Verification items for the finished model (mm, model axes). A direction names the side the tool comes from. Coordinates: 2 decimals unless noted, no trailing zeros. Write each loop counter-clockwise with the first axis right and the second up, starting at its lowest first coordinate (ties: lowest second). Pieces come first, ordered by that corner, then holes. Notation, with made-up numbers: M 74,83 L 122,83 A14 cw 122,110 Z; hole C 70.25,-13.5 d7. An arc over 180 degrees is marked long. Answer in a Markdown table with one row per item.
from build123d import *

# Parameters (mm, degrees)
SKETCH1_W             = 165.1
SKETCH1_H             = 152.4
BOSS_EXTRUDE1_DEPTH   = 12.7
BOSS_EXTRUDE2_DEPTH   = 12.7
CUT_EXTRUDE1_REACH    = 119.432
BOSS_EXTRUDE3_DEPTH   = 12.7
CUT_EXTRUDE2_DEPTH    = 12.7
F_8_CLEARANCE_HOLE1_D = 4.4958
SKETCH20_R            = 0.99187
CUT_EXTRUDE9_DEPTH    = 25.4
SKETCH21_R            = 3.175
SKETCH21_R_2          = 4.7625
CUT_EXTRUDE10_DEPTH   = 6.35


with BuildPart() as part:
    # Sketch1 → Boss-Extrude1 (new body)
    with BuildSketch(Plane.XY):
        Rectangle(SKETCH1_W, SKETCH1_H)
    extrude(amount=BOSS_EXTRUDE1_DEPTH)

    # Sketch2 → Boss-Extrude2 (add)
    with BuildSketch(Plane.XY.offset(12.7)):
        Polygon((-11.1125, 76.2), (11.1125, 76.2), (11.1125, 80.01), (10.664629469, 82.55), (-10.664629469, 82.55), (-11.1125, 80.01), align=None)
    extrude(amount=-BOSS_EXTRUDE2_DEPTH)

    # Sketch4 → Cut-Extrude1 (cut, up to next)
    with BuildSketch(Plane.XY.offset(12.7), mode=Mode.PRIVATE) as cut_extrude1_sk1:
        with BuildLine():
            Line((-17.7165, 76.2), (-11.1125, 76.2))
            ThreePointArc((-11.1125, 76.2), (-14.4145, 72.898), (-17.7165, 76.2))
        make_face()
    cut_extrude1_tool1 = extrude(cut_extrude1_sk1.sketch, amount=-CUT_EXTRUDE1_REACH, mode=Mode.PRIVATE) & part.part
    # Sketch4 → Cut-Extrude1 (cut, up to next)
    with BuildSketch(Plane.XY.offset(12.7), mode=Mode.PRIVATE) as cut_extrude1_sk2:
        with BuildLine():
            Line((11.1125, 76.2), (17.7165, 76.2))
            ThreePointArc((17.7165, 76.2), (14.4145, 72.898), (11.1125, 76.2))
        make_face()
    cut_extrude1_tool2 = extrude(cut_extrude1_sk2.sketch, amount=-CUT_EXTRUDE1_REACH, mode=Mode.PRIVATE) & part.part
    add(cut_extrude1_tool1.solids().sort_by_distance((-14.4145, 74.798588, 12.7))[0], mode=Mode.SUBTRACT)
    add(cut_extrude1_tool2.solids().sort_by_distance((14.4145, 74.798588, 12.7))[0], mode=Mode.SUBTRACT)

    # Sketch5 → Boss-Extrude3 (add)
    with BuildSketch(Plane.XY.offset(12.7)):
        Polygon((63.5, -76.2), (41.275, -76.2), (41.275, -80.01), (41.722870531, -82.55), (63.052129469, -82.55), (63.5, -80.01), align=None)
    boss_extrude3 = extrude(amount=-BOSS_EXTRUDE3_DEPTH)

    # Sketch6 → Cut-Extrude2 (cut)
    with BuildSketch(Plane.XY.offset(12.7)):
        with BuildLine():
            Line((34.671, -76.2), (41.275, -76.2))
            ThreePointArc((41.275, -76.2), (37.973, -72.898), (34.671, -76.2))
        make_face()
        with BuildLine():
            Line((63.5, -76.2), (70.104, -76.2))
            ThreePointArc((70.104, -76.2), (66.802, -72.898), (63.5, -76.2))
        make_face()
    cut_extrude2 = extrude(amount=-CUT_EXTRUDE2_DEPTH, mode=Mode.SUBTRACT)

    # Mirror1: Boss-Extrude3, Cut-Extrude2 across plane
    add(boss_extrude3.mirror(Plane(origin=(0, 0, 0), x_dir=(0, 0, 1), z_dir=(1, 0, 0))))
    add(cut_extrude2.mirror(Plane(origin=(0, 0, 0), x_dir=(0, 0, 1), z_dir=(1, 0, 0))), mode=Mode.SUBTRACT)

    # #8 Clearance Hole1 (through all)
    with Locations(Plane.XY.offset(12.7)):
        with Locations((0, -12.655936751), (63.5, 30.528732114), (-50.8, 30.528732114)):
            Hole(F_8_CLEARANCE_HOLE1_D / 2)

    # Sketch20 → Cut-Extrude9 (cut)
    with BuildSketch(Plane(origin=(82.55, 0, 0), x_dir=(0, 0, -1), z_dir=(1, 0, 0))):
        with Locations((-6.35, 0)):
            Circle(SKETCH20_R)
    cut_extrude9 = extrude(amount=-CUT_EXTRUDE9_DEPTH, mode=Mode.SUBTRACT)

    # Mirror3: Cut-Extrude9 across plane
    add(cut_extrude9.mirror(Plane(origin=(0, 0, 0), x_dir=(0, 0, 1), z_dir=(1, 0, 0))), mode=Mode.SUBTRACT)

    # Sketch21 → Cut-Extrude10 (cut)
    with BuildSketch(Plane(origin=(0, 0, 0), x_dir=(-1, 0, 0), z_dir=(0, 0, -1))):
        with Locations((0, -12.655936751)):
            Circle(SKETCH21_R)
        with Locations((-63.5, 30.528732114)):
            Circle(SKETCH21_R_2)
        with Locations((50.8, 30.528732114)):
            Circle(SKETCH21_R_2)
    extrude(amount=-CUT_EXTRUDE10_DEPTH, mode=Mode.SUBTRACT)


solid = part.part
1) Thickness scan on L1, parallel to Y at x = 71, z = 6.5; L2, parallel to Y at x = -74.5, z = 11.25; L3, parallel to Y at x = -9, z = 3.25. Record the ranges inside material, lowest first. Write a range as [from, to].
Response values:
| item | result |
|---|---|
| L1 | y = [-76.2, -0.98], [0.98, 76.2] |
| L2 | y = [-76.2, 76.2] |
| L3 | y = [-76.2, 82.55] |
2) Tool access check on faces 1 (the face through (-41.275, -78, 6)), 2 (the face through (68.258, 30.738, 3.131)), 3 (the face through (11.112, 78, 6)). Record the directions out of +Z, -Z, +X, -X, +Y, -Y that give a thin tool (end or side, any length) a straight path to the whole face; none if there is none.
Response values:
| item | result |
|---|---|
| face 1 | +Z, -Z, -Y |
| face 2 | -Z |
| face 3 | +Z, -Z, +X, +Y |
3) Release check for a two-part mould opening along X. For faces 4 (the face through (76, -76.2, 6)), 5 (the face through (63.5, -78, 6)), 6 (the face through (65.746, 30.628, 9.481)) record: +X half, -X half, draft (parallel to the pull), parting line (faces both ways), or undercut.
Response values:
| item | result |
|---|---|
| face 4 | draft |
| face 5 | +X half |
| face 6 | undercut |
4) Depth check by flat-ended pin: pin 1 (2.5 mm diameter, centred on x = 0, y = -12.66, fed in from -Z); pin 2 (1 mm diameter, centred on y = 0, z = 6.5, fed in from -X); pin 3 (1.5 mm diameter, centred on x = 9.5, z = 3, fed in from -Y); pin 4 (1.1 mm diameter, centred on y = 78, z = 8, fed in from -X). Enter the tip coordinate at first touch or a pass-through.
Response values:
| item | result |
|---|---|
| pin 1 | passes through |
| pin 2 | stops at x = -57.15 |
| pin 3 | stops at y = -76.2 |
| pin 4 | stops at x = -11.11 |
5) Sectioned sample at A-A (x = -50.8). Record the cut outline in (y, z), then the cut area to 3 significant figures.
Response values:
| item | result |
|---|---|
| outline | M -82.55,0 L 25.77,0 L 25.77,6.35 L 28.28,6.35 L 28.28,12.7 L -82.55,12.7 Z; M 32.78,6.35 L 35.29,6.35 L 35.29,0 L 76.2,0 L 76.2,12.7 L 32.78,12.7 Z |
| area | 1,930 mm² |
6) Sectioned sample at B-B (x = -25). Record the cut outline in (y, z).
Response values:
| item | result |
|---|---|
| outline | M -76.2,0 L 76.2,0 L 76.2,12.7 L -76.2,12.7 Z |
